Verification items for the finished model (mm, model axes). A direction names the side the tool comes from. Give positions to 0.01 mm unless a question says otherwise; leave off trailing zeros. Loops run counter-clockwise (first coordinate to the right, second up) from the corner with the lowest first, then second, coordinate; pieces in that order, holes last. Notation, with made-up numbers: (27.25, -25.75) - (69.25, -25.75) arc R19 ccw to (69.25, 11.25) - close; hole circle Ø5 at (65.5, 46.25). An arc over 180 degrees is marked (long way). Answer in a Markdown table with one row per item.
```python
from build123d import *

# Parameters (mm, degrees)
BOSS_EXTRUDE1_DEPTH                               = 3.175
SKETCH4_W                                         = 7.1374
SKETCH4_H                                         = 3.175
F_4_CLEARANCE_HOLE1_D                             = 3.3
F_4_CLEARANCE_HOLE1_DEPTH                         = 3.175
CSK_FOR_4_FLAT_HEAD_MACHINE_SCREW_100_D           = 3.4
CSK_FOR_4_FLAT_HEAD_MACHINE_SCREW_100_DEPTH       = 3.175
CSK_FOR_4_FLAT_HEAD_MACHINE_SCREW_100_CSINK_D     = 6.3
CSK_FOR_4_FLAT_HEAD_MACHINE_SCREW_100_CSINK_ANGLE = 90
CUT_EXTRUDE1_DEPTH                                = 4.175


with BuildPart() as part:
    # Sketch1 → Boss-Extrude1 (new body)
    with BuildSketch(Plane.XY.offset(3.175)):
        with BuildLine():
            Line((53.959502015, 32.443258315), (22.445653919, 38))
            Line((22.445653919, 38), (0, 38))
            ThreePointArc((0, 38), (-32.908965344, -19), (32.908965344, -19))
            Line((32.908965344, -19), (54.559600438, 18.5))
            ThreePointArc((54.559600438, 18.5), (56.289246799, 25.558984429), (53.959502015, 32.443258315))
        make_face()
    extrude(amount=-BOSS_EXTRUDE1_DEPTH)

    # Sketch4 → Cut-Revolve1 (revolve, cut)
    with BuildSketch(Plane.XZ):
        with Locations((3.5687, 1.5875)):
            Rectangle(SKETCH4_W, SKETCH4_H)
    revolve(axis=Axis((0, 0, 3.175), (0, 0, -1)), mode=Mode.SUBTRACT)

    # #4 Clearance Hole1
    with Locations(Plane.XY.offset(3.175)):
        with Locations((18.5, 0), (0, -18.5), (-18.5, 0), (0, 18.5)):
            Hole(F_4_CLEARANCE_HOLE1_D / 2, depth=F_4_CLEARANCE_HOLE1_DEPTH)

    # CSK for #4 Flat Head Machine Screw (100)1
    with Locations(Plane.XY.offset(3.175)):
        with Locations((-9.959292144, 5.75), (-9.959292144, -5.75), (0, -11.5), (9.959292144, -5.75), (9.959292144, 5.75), (0, 11.5)):
            CounterSinkHole(CSK_FOR_4_FLAT_HEAD_MACHINE_SCREW_100_D / 2, CSK_FOR_4_FLAT_HEAD_MACHINE_SCREW_100_CSINK_D / 2, depth=CSK_FOR_4_FLAT_HEAD_MACHINE_SCREW_100_DEPTH, counter_sink_angle=CSK_FOR_4_FLAT_HEAD_MACHINE_SCREW_100_CSINK_ANGLE)

    # Sketch9 → Cut-Extrude1 (cut, through all)
    with BuildSketch(Plane(origin=(0, 0, 0), x_dir=(-1, 0, 0), z_dir=(0, 0, -1))):
        Polygon((-2.364186438, -9.09489103), (-6.694313457, -6.59489103), (-5.439804269, -4.422017377), (-1.10967725, -6.922017377), align=None)
    extrude(amount=-CUT_EXTRUDE1_DEPTH, mode=Mode.SUBTRACT)


solid = part.part
```
Q1. Draft check along X on faces 3 (the face through (43.583, -0.513, 1.61)), 4 (the face through (11, 38, 2)), 5 (the face through (1.76, -8.05, 1.57)). Enter one of: +X half, -X half, draft (parallel to the pull), parting line (faces both ways), or undercut.
Completed:
| item | result |
|---|---|
| face 3 | +X half |
| face 4 | draft |
| face 5 | undercut |
Q2. Sectioned sample at C-C (y = 5.75). Record the cut outline in (x, z) (3 decimals).
Completed:
| item | result |
|---|---|
| outline | (-37.562, 0) - (-11.659, 0) - (-11.659, 1.725) - (-13.109, 3.175) - (-37.562, 3.175) - close; (-8.259, 0) - (-4.228, 0) - (-4.228, 3.175) - (-6.809, 3.175) - (-8.259, 1.725) - close; (4.228, 0) - (8.259, 0) - (8.259, 1.725) - (6.809, 3.175) - (4.228, 3.175) - close; (11.659, 0) - (47.198, 0) - (47.198, 3.175) - (13.109, 3.175) - (11.659, 1.725) - close |
Q3. Sectioned sample at B-B (y = -11.5). Record the cut outline in (x, z) (3 decimals), and give its area (3 significant figures).
Completed:
| item | result |
|---|---|
| outline | (-36.218, 0) - (-1.7, 0) - (-1.7, 1.725) - (-3.15, 3.175) - (-36.218, 3.175) - close; (1.7, 0) - (37.239, 0) - (37.239, 3.175) - (3.15, 3.175) - (1.7, 1.725) - close |
| area | 220 mm^2 |
Q4. Go/stop test with flat-tipped pins: P1, Ø4.5, axis at x = 9.96, y = 5.75, coming from the +Z side; P2, Ø5.5, axis at x = 0, y = 11.5, coming from the +Z side (3 decimals); P3, Ø1, axis at y = 18, z = 0.5, coming from the +X side. Record where each tip stops, or that it passes through.
Completed:
| item | result |
|---|---|
| P1 | z = 2.28 |
| P2 | z = 2.775 |
| P3 | x = 54.56 |
Q5. Thickness scan on line 1 (Y direction, x = 10.5, z = 0.55); line 2 (Y direction, x = 11.5, z = 2.9); line 3 (X direction, y = 5.75, z = 0.4). Record the ranges inside material, lowest first.
Completed:
| item | result |
|---|---|
| line 1 | -36.52 to -7.36, -4.14 to 4.14, 7.36 to 38 |
| line 2 | -36.22 to -8.18, -3.32 to 3.32, 8.18 to 38 |
| line 3 | -37.56 to -11.66, -8.26 to -4.23, 4.23 to 8.26, 11.66 to 47.2 |
Q6. Sectioned sample at A-A (z = 0.8). Give the number of separate pieces and of enclosed holes in the cut face, and give its area (3 significant figures).
Completed:
| item | result |
|---|---|
| separate pieces | 1 |
| enclosed holes | 11 |
| area | 5,080 mm^2 |
Q7. Tool access check on faces 1 (the face through (8, 1, 0)), 2 (the face through (4.5, -7.86, 1.57)). Record the directions out of +Z, -Z, +X, -X, +Y, -Y that give a thin tool (end or side, any length) a straight path to the whole face; none if there is none.
Completed:
| item | result |
|---|---|
| face 1 | -Z, +X, -X, +Y, -Y |
| face 2 | +Z, -Z |
Q8. Sectioned sample at D-D (x = -18.5). Record the cut outline in (y, z) (3 decimals), and give its area (3 significant figures).
Completed:
| item | result |
|---|---|
| outline | (-33.193, 0) - (-1.65, 0) - (-1.65, 3.175) - (-33.193, 3.175) - close; (1.65, 0) - (33.193, 0) - (33.193, 3.175) - (1.65, 3.175) - close |
| area | 200 mm^2 |
